Can you work these out from the model? Positions are in its coordinate system, mm. A direction names the side the tool comes from. Round coordinates to 2 decimals unless told otherwise and drop trailing zeros. Write each loop counter-clockwise with the first axis right and the second up, starting at its lowest first coordinate (ties: lowest second). Pieces come first, ordered by that corner, then holes. Notation, with made-up numbers: (60, -34.75) -> (106, -34.75) arc R17 ccw to (106, -18.75) -> close; hole circle Ø7 at (80.25, 58). An arc over 180 degrees is marked (long way). Write item = value, one per line. Start each with the question number.
1) Imagine slicing it at C-C, the plane x = 13. Please give me the cut outline in (y, z).
2) Thinking about a two-plate mould opening in X: for faces 1 (the face through (1.021, -23.577, 1.038)), 2 (the face through (2.5, -13, -20)), 3 (the face through (-2.5, -13.4, -15.3)), 4 (the face through (17.605, 3.592, -19.139)), which applies, +X half, -X half, draft (parallel to the pull), parting line (faces both ways), or undercut?
3) I'm going to push flat-ended pins straight in: pin 1 (0.6 mm diameter, centred on x = 22, z = -9.5, fed in from -Y); pin 2 (1.5 mm diameter, centred on x = 4, y = 8, fed in from -Z); pin 3 (3 mm diameter, centred on x = 23, z = -12.5, fed in from +Y). Where does each tip first touch, or does it pass through?
4) Imagine slicing it at D-D, the plane z = 22. Please give me the cut outline in (x, y), then the cut area to 3 significant figures.
5) Imagine slicing it at B-B, the plane y = 4. Please give me the cut outline in (x, z), then the cut area to 3 significant figures.
6) If I drill on line 1 (X direction, y = 1.5, z = 24.5); line 2 (Z direction, x = 19.5, y = 0); line 3 (Z direction, x = 21.75, y = 0), over which ranges is the centre line in solid material (lowest first)?
7) Imagine slicing it at A-A, the plane z = 0. Please give me the cut outline in (x, y).
8) For faces 5 (the face through (25, -6, 0)), 6 (the face through (-1.486, -20.633, -15.821)), 7 (the face through (22, 1, -10.4)), 8 (the face through (17.605, 3.562, 19.115)), 9 (the face through (20, 13, -20)), which set-ups out of +Z, -Z, +X, -X, +Y, -Y let a thin tool reach every point of the face, with its end or its side?
from build123d import *

# Parameters (mm, degrees)
EXTRUSION1_DEPTH = 28.5
EXTRUSION2_DEPTH = 6


with BuildPart() as part:
    # Esquisse1 → Révolution1 (revolve)
    with BuildSketch(Plane.XY):
        Polygon((-2.5, 20), (-2.5, 26), (-0.5, 26), (-0.5, 23.6), (2.5, 23.6), (2.5, 30), (20, 30), (20, 23.6), (23, 23.6), (23, 26), (25, 26), (25, 4), (10, 4), (10, 20), align=None)
    revolve(axis=Axis((10, 0, 0), (1, 0, 0)))

    # Esquisse2 → Extrusion1 (cut, through all)
    with BuildSketch(Plane(origin=(25, 0, 0), x_dir=(0, 0, -1), z_dir=(1, 0, 0))):
        with BuildLine():
            Line((17.944358445, 3), (-17.944358445, 3))
            ThreePointArc((-17.944358445, 3), (-19.127003214, 3.577312972), (-19.399306427, 4.864864865))
            ThreePointArc((-19.399306427, 4.864864865), (0, 20), (19.399306427, 4.864864865))
            ThreePointArc((19.399306427, 4.864864865), (19.127003214, 3.577312972), (17.944358445, 3))
        make_face()
    extrude(amount=-EXTRUSION1_DEPTH, mode=Mode.SUBTRACT)

    # Esquisse3 → Extrusion2 (cut)
    with BuildSketch(Plane(origin=(25, 0, 0), x_dir=(0, 0, -1), z_dir=(1, 0, 0))):
        with BuildLine():
            Line((-10.4, -1.829201479), (-10.4, 3.170798521))
            Line((-10.4, 3.170798521), (-13.6, 3.170798521))
            Line((-13.6, 3.170798521), (-13.6, -1.829201479))
            Line((-13.6, -1.829201479), (-15.5, -1.829201479))
            ThreePointArc((-15.5, -1.829201479), (-16.560660172, -2.268541307), (-17, -3.329201479))
            Line((-17, -3.329201479), (-17, -3.829201479))
            ThreePointArc((-17, -3.829201479), (-16.560660172, -4.889861651), (-15.5, -5.329201479))
            Line((-15.5, -5.329201479), (-8.5, -5.329201479))
            ThreePointArc((-8.5, -5.329201479), (-7.439339828, -4.889861651), (-7, -3.829201479))
            Line((-7, -3.829201479), (-7, -3.329201479))
            ThreePointArc((-7, -3.329201479), (-7.439339828, -2.268541307), (-8.5, -1.829201479))
            Line((-8.5, -1.829201479), (-10.4, -1.829201479))
        make_face()
        with BuildLine():
            Line((7, -3.329201479), (7, -3.829201479))
            ThreePointArc((7, -3.829201479), (7.439339828, -4.889861651), (8.5, -5.329201479))
            Line((8.5, -5.329201479), (15.5, -5.329201479))
            ThreePointArc((15.5, -5.329201479), (16.560660172, -4.889861651), (17, -3.829201479))
            Line((17, -3.829201479), (17, -3.329201479))
            ThreePointArc((17, -3.329201479), (16.560660172, -2.268541307), (15.5, -1.829201479))
            Line((15.5, -1.829201479), (13.6, -1.829201479))
            Line((13.6, -1.829201479), (13.6, 3.170798521))
            Line((13.6, 3.170798521), (10.4, 3.170798521))
            Line((10.4, 3.170798521), (10.4, -1.829201479))
            Line((10.4, -1.829201479), (8.5, -1.829201479))
            ThreePointArc((8.5, -1.829201479), (7.439339828, -2.268541307), (7, -3.329201479))
        make_face()
    extrude(amount=-EXTRUSION2_DEPTH, mode=Mode.SUBTRACT)


solid = part.part
Reported:
q1.outline = circle Ø60 at (0, 0); hole (3, -17.94) arc R1.5 ccw to (4.86, -19.4) arc R20 ccw to (4.86, 19.4) arc R1.5 ccw to (3, 17.94) -> (3, 2.65) arc R4 ccw (long way) to (3, -2.65) -> close
q2.face_1 = undercut
q2.face_2 = undercut
q2.face_3 = -X half
q2.face_4 = draft
q3.pin_1 = -21.73
q3.pin_2 = -29.11
q3.pin_3 = 23.56
q4.outline = (-2.5, -13.86) -> (-0.5, -13.86) -> (-0.5, -8.54) -> (2.5, -8.54) -> (2.5, -20.4) -> (20, -20.4) -> (20, -8.54) -> (23, -8.54) -> (23, -13.86) -> (25, -13.86) -> (25, 13.86) -> (23, 13.86) -> (23, 8.54) -> (20, 8.54) -> (20, 20.4) -> (2.5, 20.4) -> (2.5, 8.54) -> (-0.5, 8.54) -> (-0.5, 13.86) -> (-2.5, 13.86) -> close
q4.area = 927 mm²
q5.outline = (-2.5, -25.69) -> (-0.5, -25.69) -> (-0.5, -23.26) -> (2.5, -23.26) -> (2.5, -29.73) -> (20, -29.73) -> (20, -23.26) -> (23, -23.26) -> (23, -25.69) -> (25, -25.69) -> (25, -19.36) -> (10, -19.36) -> (10, -19.6) -> (-2.5, -19.6) -> close; (-2.5, 19.6) -> (10, 19.6) -> (10, 19.36) -> (25, 19.36) -> (25, 25.69) -> (23, 25.69) -> (23, 23.26) -> (20, 23.26) -> (20, 29.73) -> (2.5, 29.73) -> (2.5, 23.26) -> (-0.5, 23.26) -> (-0.5, 25.69) -> (-2.5, 25.69) -> close
q5.area = 455 mm²
q6.line_1 = -2.5 to -0.5, 2.5 to 20, 23 to 25
q6.line_2 = -30 to -13.6, -10.4 to -4, 4 to 10.4, 13.6 to 30
q6.line_3 = -23.6 to -13.6, -10.4 to -4, 4 to 10.4, 13.6 to 23.6
q7.outline = (-2.5, -26) -> (-0.5, -26) -> (-0.5, -23.6) -> (2.5, -23.6) -> (2.5, -30) -> (20, -30) -> (20, -23.6) -> (23, -23.6) -> (23, -26) -> (25, -26) -> (25, -4) -> (10, -4) -> (10, -20) -> (-2.5, -20) -> close; (-2.5, 20) -> (25, 20) -> (25, 26) -> (23, 26) -> (23, 23.6) -> (20, 23.6) -> (20, 30) -> (2.5, 30) -> (2.5, 23.6) -> (-0.5, 23.6) -> (-0.5, 26) -> (-2.5, 26) -> close
q8.face_5 = +Z, -Z, +X, +Y, -Y
q8.face_6 = -X
q8.face_7 = +X
q8.face_8 = +X, -X
q8.face_9 = none
